For this review, take the finished solid that the model builds, in its own axes (mm). Round coordinates to 2 decimals unless told otherwise and drop trailing zeros. Write each loop counter-clockwise with the first axis right and the second up, starting at its lowest first coordinate (ties: lowest second). Pieces come first, ordered by that corner, then holes. Notation, with made-up numbers: (80, -24.5) -> (94, -24.5) arc R21 ccw to (94, 4.5) -> close; hole circle Ø7 at (4.5, 29). An arc over 180 degrees is marked (long way). Write each question's results on one line, items separated by ' | '. Start each with the question number.
Item 1: Add section A-A (z = 332). State the section outline as (x, y) points.
Item 2: To check wall thickness, follow line 1 along Y through (x, z) = (-4, 15); line 2 along Z through (x, y) = (-20, -18.5); line 3 along X through (y, z) = (9.5, 147). State the ranges of each line that lie inside material, in increasing order.
Item 3: Add section B-B (y = 8). State the section outline as (x, z) points, plus the area to 3 significant figures.
Item 4: Clearance check with flat-ended pins moving along their axes: pin 1 (3.5 mm diameter, centred on y = -3, z = 585, fed in from -X); pin 2 (1 mm diameter, centred on x = -37, y = -7, fed in from -Z); pin 3 (10.5 mm diameter, centred on x = -28, y = -4, fed in from +Z). State where each tip first meets the part, or that it passes through.
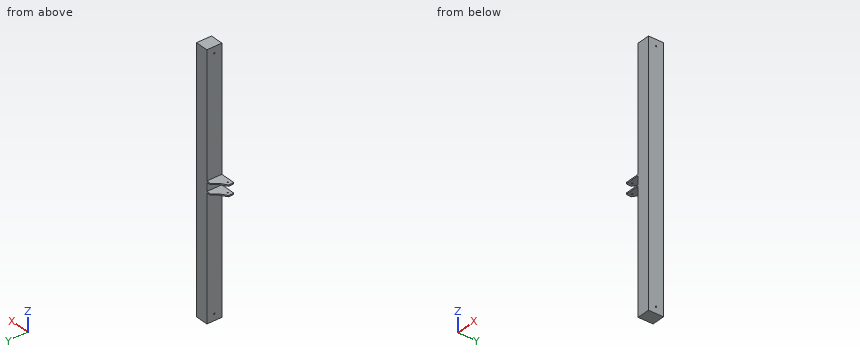
Autodesk Inventor part; units mm, degrees
ref_plane "YZ Plane" through (0, 0, 0) normal (1, 0, 0) x (0, 1, 0)
ref_plane "XZ Plane" through (0, 0, 0) normal (0, 1, 0) x (-1, 0, 0)
ref_plane "XY Plane" through (0, 0, 0) normal (0, 0, 1) x (1, 0, 0)
sketch "Skizze1" plane through (0, 0, 0) normal (0, 0, 1) x (1, 0, 0)
  line L0 (-65.5041, 0) -> (25.4959, 0)
  line L1 (0, -27.5001) -> (0, 21.4999)
  line L2 (-17.5041, 14.4999) -> (12.4959, 14.4999)
  line L3 (12.4959, 14.4999) -> (12.4959, -20.5001)
  line L4 (12.4959, -20.5001) -> (-17.5041, -20.5001)
  line L5 (-17.5041, -20.5001) -> (-17.5041, 14.4999)
  point P0 (0, 0)
  dimension "d0" = 30
  dimension "d1" = 35
extrude "Extrusion1" add sketch "Skizze1" along normal blind 600
sketch "Skizze2" plane through (-17.5041, -20.5001, 0) normal (-1, 0, 0) x (0, 0, 1)
  line L0 (0, 0) -> (600, 0)
  line L1 (287, 35) -> (290, 35)
  line L2 (290, 35) -> (290, 0)
  line L3 (290, 0) -> (287, 0)
  line L4 (287, 0) -> (287, 35)
  line L5 (0, 35) -> (600, 35)
  line L6 (310, 35) -> (313, 35)
  line L7 (313, 35) -> (313, 0)
  line L8 (313, 0) -> (310, 0)
  line L9 (310, 0) -> (310, 35)
  line L10 (600, 35) -> (600, 0)
  point P0 (0, 20.5001)
  point P1 (310, 0)
  point P2 (313, 0)
  point P3 (287, 0)
  dimension "d4" = 287
  dimension "d5" = 3
  dimension "d6" = 20
  dimension "d7" = 3
  dimension "d10" = 35
extrude "Extrusion2" add sketch "Skizze2" along normal blind 35 contours L4 L1 L2 L0 | L9 L5 L7 L0
sketch "Skizze3" plane through (-17.5041, -20.5001, 313) normal (0, 0, 1) x (1, 0, 0)
  line L0 (0, 35) -> (-35, 35)
  line L1 (-10, 35) -> (-20, 22.6396)
  line L2 (-20, 22.6396) -> (-35, 12.5)
  line L3 (-35, 12.5) -> (-35, 35)
  line L4 (-35, 35) -> (-10, 35)
  point P0 (17.5041, 20.5001)
  dimension "d11" = 25
  dimension "d12" = 15
  dimension "d13" = 22.5
extrude "Extrusion3" cut sketch "Skizze3" against normal blind 50
fillet "Rundung1" radius 2 4 edges at (-52.5041, -8.0001, 288.5) (-52.5041, -8.0001, 311.5) (-52.5041, -20.5001, 288.5) (-52.5041, -20.5001, 311.5)
sketch "Skizze4" plane through (-17.5041, -20.5001, 313) normal (0, 0, 1) x (1, 0, 0)
  line L0 (-35, 2) -> (-35, 11.4379)
  line L1 (0, 0) -> (-33, 0)
  point P0 (17.5041, 20.5001)
  point P1 (-27, 8)
  dimension "d17" = 8
  dimension "d18" = 8
hole "Bohrung1" at (-44.5041, -12.5001, 313) direction (0, 0, -1) diameter 3 end through all
sketch "Skizze5" plane through (-17.5041, -20.5001, 600) normal (-1, 0, 0) x (0, 0, 1)
  line L0 (0, 35) -> (0, 0)
  line L1 (-600, 35) -> (-600, 0)
  line L2 (-600, 35) -> (-313, 35)
  line L3 (-287, 35) -> (0, 35)
  point P0 (-600, 20.5001)
  point P1 (-585, 17.5)
  point P2 (-15, 17.5)
  dimension "d26" = 15
  dimension "d27" = 15
  dimension "d28" = 17.5
  dimension "d29" = 17.5
hole "Bohrung2" at (-17.5041, -3.0001, 15) at (-17.5041, -3.0001, 585) direction (1, 0, 0) diameter 3 depth 30 tip angle 118
properties part number "träger hinten mit motorhalterung" material "Stahl"
Responses:
1) outline: (-17.5, -20.5) -> (12.5, -20.5) -> (12.5, 14.5) -> (-17.5, 14.5) -> close
2) line 1: y = -20.5 to -4.5, -1.5 to 14.5 | line 2: z = 287 to 290, 310 to 313 | line 3: x = -17.5 to 12.5
3) outline: (-32.76, 287) -> (-17.5, 287) -> (-17.5, 0) -> (12.5, 0) -> (12.5, 600) -> (-17.5, 600) -> (-17.5, 313) -> (-32.76, 313) -> (-32.76, 310) -> (-17.5, 310) -> (-17.5, 290) -> (-32.76, 290) -> close | area: 18,100 mm^2
4) pin 1: stops at x = -17.5 | pin 2: stops at z = 287 | pin 3: stops at z = 313
